from build123d import *

# Parameters (mm, degrees)
SKETCH_2_W      = 10
SKETCH_2_H      = 10
EXTRUDE_1_DEPTH = 20
FILLET_1_R      = 2
CHAMFER_1_SIZE  = 1
CHAMFER_2_SIZE  = 1
CHAMFER_2_SIZE2 = 0.577350269


with BuildPart() as part:
    # Эскиз1 → Повернуть1 (revolve)
    with BuildSketch(Plane.XY, mode=Mode.PRIVATE) as revolve_1_sk:
        Polygon((0, 0), (0, -10.5), (25, -10.5), (25, -9), (42, -9), (42, -7.5), (65, -7.5), (65, 0), align=None)
    revolve(revolve_1_sk.sketch.rotate(Axis((0, 0, 0), (1, 0, 0)), 270), axis=Axis((0, 0, 0), (1, 0, 0)))

    # Эскиз2 → Бобышка-Вытянуть1 (add)
    with BuildSketch(Plane.ZY):
        Rectangle(SKETCH_2_W, SKETCH_2_H)
    extrude(amount=EXTRUDE_1_DEPTH)

    # Скругление1
    fillet_1_edges = [part.edges().sort_by_distance(p)[0] for p in [
        (0, 0, -10.5),
    ]]
    fillet(fillet_1_edges, radius=FILLET_1_R)

    # Фаска1
    chamfer_1_edges = [part.edges().sort_by_distance(p)[0] for p in [
        (25, 0, -10.5),
    ]]
    chamfer(chamfer_1_edges, length=CHAMFER_1_SIZE)

    # Фаска2
    chamfer_2_edges = [part.edges().sort_by_distance(p)[0] for p in [
        (42, 0, -9),
    ]]
    chamfer_2_side = [part.faces().sort_by_distance(p)[0] for p in [
        (42, 0, -8.745441559),
    ]]
    chamfer(chamfer_2_edges, length=CHAMFER_2_SIZE, length2=CHAMFER_2_SIZE2, reference=chamfer_2_side[0])


solid = part.part
Input: part model. Units: mm. Frame: model coordinates. A direction names the side the tool comes from. Give positions to 0.01 mm unless a question says otherwise; leave off trailing zeros. Order: outer loops, then holes, each group sorted by start corner. A loop starts at its lowest first (then second) coordinate and runs counter-clockwise, first axis right, second up. Notation, with made-up numbers: (-6, -37) -> (34, -37) arc R23 ccw to (34, 0) -> close; hole circle Ø7 at (-30, 9). An arc over 180 degrees is marked (long way). Use one line per item in the form item = value.
1) Section A-A, the plane z = 0. Return loops of the section in (x, y).
Response values:
outline = (-20, -5) -> (0, -5) -> (0, -8.5) arc R2 ccw to (2, -10.5) -> (24, -10.5) -> (25, -9.5) -> (25, -9) -> (41.42, -9) -> (42, -8) -> (42, -7.5) -> (65, -7.5) -> (65, 7.5) -> (42, 7.5) -> (42, 8) -> (41.42, 9) -> (25, 9) -> (25, 9.5) -> (24, 10.5) -> (2, 10.5) arc R2 ccw to (0, 8.5) -> (0, 5) -> (-20, 5) -> close
2) Section D-D, the plane x = 30.5. Return loops of the section in (y, z).
Response values:
outline = circle Ø18 at (0, 0)
3) Section C-C, the plane x = -4.5. Return loops of the section in (y, z), and give its area (3 significant figures).
Response values:
outline = (-5, -5) -> (5, -5) -> (5, 5) -> (-5, 5) -> close
area = 100 mm^2
4) First-contact query: pin 1 Ø1 at (x, z) = (10, -3.5) entering from +Y; pin 2 Ø11 at (x, y) = (-14.5, 1) entering from +Z; pin 3 Ø5 at (x, y) = (40.5, -5) entering from +Z. Flat tips, straight axial feed; report the tip coordinate or a pass-through.
Response values:
pin_1 = 10.06
pin_2 = 5
pin_3 = 8.65
5) Reachability of faces 4 (the cylindrical face through (33.326, -2.703, 8.584)), 5 (the flat face through (-10, 0, -5)), 6 (the flat face through (-10, -5, 0)), 7 (the flat face through (-10, 5, 0)), 8 (the cylindrical face through (13.2, -3.2, 10)) from +Z, -Z, +X, -X, +Y, -Y: full face, straight path, thin tool, end or side. Return the list, or none.
Response values:
face_4 = +X
face_5 = -Z, -X, +Y, -Y
face_6 = +Z, -Z, -X, -Y
face_7 = +Z, -Z, -X, +Y
face_8 = +X, -X
6) Line query: probe 1 along Z at (x, y) = (-3, -2.75); probe 2 along X at (y, z) = (7, 1.75). Output: solid intervals per line, ascending.
Response values:
probe_1 = -5 to 5
probe_2 = 0 to 65
7) Mould query, pull axis Z, two halves, no side actions, for faces 1 (the flat face through (0, 6, 0)), 2 (the flat face through (-10, 0, 5)), 3 (the cylindrical face through (53.661, -0.33, -7.493)). Classes: pulls with the +Z half, pulls with the -Z half, needs draft (parallel to the pull), parting line crosses it, or undercut.
Response values:
face_1 = needs draft
face_2 = pulls with the +Z half
face_3 = parting line crosses it
